Verification items for the finished model (mm, model axes). Round coordinates to 2 decimals unless told otherwise and drop trailing zeros. Write each loop counter-clockwise with the first axis right and the second up, starting at its lowest first coordinate (ties: lowest second). Pieces come first, ordered by that corner, then holes. Notation, with made-up numbers: (79.25, -14) -> (104.25, -14) arc R14 cw to (104.25, 5) -> close; hole circle Ø6 at (61, 29.25). An arc over 180 degrees is marked (long way). Answer as a JSON object with one key per item and string values. Group by question number.
(1) Sectioned sample at A-A on x = -25. Record the cut outline in (y, z).
(2) Gauge pin test, flat ends, axial feed: pin 1 Ø1.5 at (x, z) = (-21, 3.5) entering from -Y; pin 2 Ø1 at (x, z) = (25, 1) entering from -Y; pin 3 Ø2 at (y, z) = (64.5, 4) entering from -X. Record the tip position at first contact, or that the pin passes through.
(3) Scan lines: L1, parallel to Y at x = -17.5, z = 3.1; L2, parallel to X at y = 78, z = 2.75; L3, parallel to Y at x = -4, z = 0.3. Record each from-to range of solid material in increasing order. Write a range as from..to.
(4) Sectioned sample at C-C on x = -12.5. Record the cut outline in (y, z), and give its area (3 significant figures).
(5) Sectioned sample at B-B on y = 82. Record the cut outline in (x, z), and give its area (3 significant figures).
(6) Sectioned sample at D-D on z = 2.6. Count the separate pieces of the cut face and the enclosed holes in it, and give its area (3 significant figures).
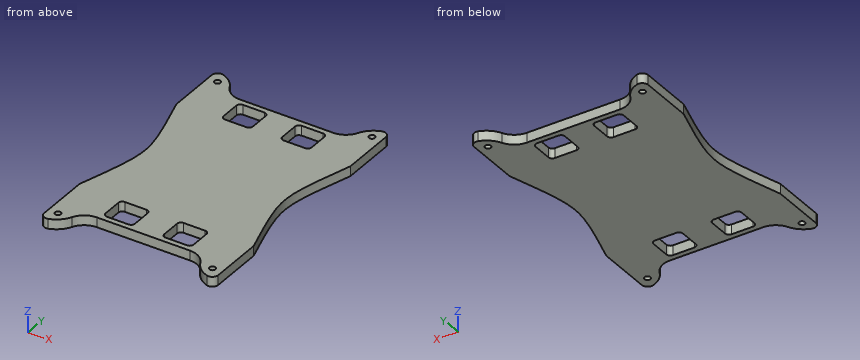
```python
from build123d import *

# Parameters (mm, degrees)
RESSALTO_EXTRUS_O3_DEPTH = 5
ESBO_O4_R                = 1.5
CORTE_EXTRUS_O3_DEPTH    = 10


with BuildPart() as part:
    # Esboço1 → Ressalto-extrusão3 (new body)
    with BuildSketch(Plane.XY):
        with BuildLine():
            Line((-31.851570772, -17.801096987), (-27.063885949, -17.801096987))
            Line((-27.063885949, -17.801096987), (10.936114051, -17.801096987))
            Line((10.936114051, -17.801096987), (15.723798874, -17.801096987))
            ThreePointArc((15.723798874, -17.801096987), (21.039894205, -19.331201448), (24.729153299, -23.4532709))
            ThreePointArc((24.729153299, -23.4532709), (27.934250919, -27.635644423), (32.536114051, -30.202306605))
            ThreePointArc((32.536114051, -30.202306605), (35.210937986, -29.759166326), (36.436114051, -27.340489001))
            Line((36.436114051, -27.340489001), (36.436114051, -17.801096987))
            Line((36.436114051, -17.801096987), (36.436114051, 0.198903013))
            add(Edge.make_bspline(
                [(36.436114051, 75.398903013), (24.729153299, 37.798903013), (36.436114051, 0.198903013)],
                knots=[0, 0, 0, 1, 1, 1], degree=2, weights=[1, 3, 1]))
            Line((36.436114051, 75.398903013), (36.436114051, 93.398903013))
            Line((36.436114051, 93.398903013), (36.436114051, 102.938295027))
            ThreePointArc((36.436114051, 102.938295027), (35.210937986, 105.356972352), (32.536114051, 105.800112631))
            ThreePointArc((32.536114051, 105.800112631), (27.934250919, 103.23345045), (24.729153299, 99.051076926))
            ThreePointArc((24.729153299, 99.051076926), (21.039894205, 94.929007474), (15.723798874, 93.398903013))
            Line((15.723798874, 93.398903013), (10.936114051, 93.398903013))
            Line((10.936114051, 93.398903013), (-27.063885949, 93.398903013))
            Line((-27.063885949, 93.398903013), (-31.851570772, 93.398903013))
            ThreePointArc((-31.851570772, 93.398903013), (-37.167666102, 94.929007474), (-40.856925197, 99.051076926))
            ThreePointArc((-40.856925197, 99.051076926), (-44.062022817, 103.23345045), (-48.663885949, 105.800112631))
            ThreePointArc((-48.663885949, 105.800112631), (-51.338709884, 105.356972352), (-52.563885949, 102.938295027))
            Line((-52.563885949, 102.938295027), (-52.563885949, 93.398903013))
            Line((-52.563885949, 93.398903013), (-52.563885949, 75.398903013))
            add(Edge.make_bspline(
                [(-52.563885949, 75.398903013), (-40.856925197, 37.798903013), (-52.563885949, 0.198903013)],
                knots=[0, 0, 0, 1, 1, 1], degree=2, weights=[1, 3, 1]))
            Line((-52.563885949, 0.198903013), (-52.563885949, -17.801096987))
            Line((-52.563885949, -17.801096987), (-52.563885949, -27.340489001))
            ThreePointArc((-52.563885949, -27.340489001), (-51.338709884, -29.759166326), (-48.663885949, -30.202306605))
            ThreePointArc((-48.663885949, -30.202306605), (-44.062022817, -27.635644423), (-40.856925197, -23.4532709))
            ThreePointArc((-40.856925197, -23.4532709), (-37.167666102, -19.331201448), (-31.851570772, -17.801096987))
        make_face()
    extrude(amount=RESSALTO_EXTRUS_O3_DEPTH)

    # Esboço4 → Corte-extrusão3 (cut)
    with BuildSketch(Plane(origin=(0, 0, 0), x_dir=(-1, 0, 0), z_dir=(0, 0, -1))):
        with Locations((-31.436114051, 99.800112631)):
            Circle(ESBO_O4_R)
        with Locations((47.563885949, 99.800112631)):
            Circle(ESBO_O4_R)
        with Locations((47.563885949, -24.202306605)):
            Circle(ESBO_O4_R)
        with Locations((-31.436114051, -24.202306605)):
            Circle(ESBO_O4_R)
        with BuildLine():
            Line((-12.436114051, 90.598903013), (-1.436114051, 90.598903013))
            ThreePointArc((-1.436114051, 90.598903013), (-0.021900489, 90.013116575), (0.563885949, 88.598903013))
            Line((0.563885949, 88.598903013), (0.563885949, 78.698903013))
            ThreePointArc((0.563885949, 78.698903013), (-0.021900489, 77.284689451), (-1.436114051, 76.698903013))
            Line((-1.436114051, 76.698903013), (-12.436114051, 76.698903013))
            ThreePointArc((-12.436114051, 76.698903013), (-13.850327613, 77.284689451), (-14.436114051, 78.698903013))
            Line((-14.436114051, 78.698903013), (-14.436114051, 88.598903013))
            ThreePointArc((-14.436114051, 88.598903013), (-13.850327613, 90.013116575), (-12.436114051, 90.598903013))
        make_face()
        with BuildLine():
            Line((17.563885949, 90.598903013), (28.563885949, 90.598903013))
            ThreePointArc((28.563885949, 90.598903013), (29.978099511, 90.013116575), (30.563885949, 88.598903013))
            Line((30.563885949, 88.598903013), (30.563885949, 78.698903013))
            ThreePointArc((30.563885949, 78.698903013), (29.978099511, 77.284689451), (28.563885949, 76.698903013))
            Line((28.563885949, 76.698903013), (17.563885949, 76.698903013))
            ThreePointArc((17.563885949, 76.698903013), (16.149672387, 77.284689451), (15.563885949, 78.698903013))
            Line((15.563885949, 78.698903013), (15.563885949, 88.598903013))
            ThreePointArc((15.563885949, 88.598903013), (16.149672387, 90.013116575), (17.563885949, 90.598903013))
        make_face()
        with BuildLine():
            Line((30.563885949, -13.001096987), (30.563885949, -3.101096987))
            ThreePointArc((30.563885949, -3.101096987), (29.978099511, -1.686883425), (28.563885949, -1.101096987))
            Line((28.563885949, -1.101096987), (17.563885949, -1.101096987))
            ThreePointArc((17.563885949, -1.101096987), (16.149672387, -1.686883425), (15.563885949, -3.101096987))
            Line((15.563885949, -3.101096987), (15.563885949, -13.001096987))
            ThreePointArc((15.563885949, -13.001096987), (16.149672387, -14.415310549), (17.563885949, -15.001096987))
            Line((17.563885949, -15.001096987), (28.563885949, -15.001096987))
            ThreePointArc((28.563885949, -15.001096987), (29.978099511, -14.415310549), (30.563885949, -13.001096987))
        make_face()
        with BuildLine():
            Line((0.563885949, -13.001096987), (0.563885949, -3.101096987))
            ThreePointArc((0.563885949, -3.101096987), (-0.021900489, -1.686883425), (-1.436114051, -1.101096987))
            Line((-1.436114051, -1.101096987), (-12.436114051, -1.101096987))
            ThreePointArc((-12.436114051, -1.101096987), (-13.850327613, -1.686883425), (-14.436114051, -3.101096987))
            Line((-14.436114051, -3.101096987), (-14.436114051, -13.001096987))
            ThreePointArc((-14.436114051, -13.001096987), (-13.850327613, -14.415310549), (-12.436114051, -15.001096987))
            Line((-12.436114051, -15.001096987), (-1.436114051, -15.001096987))
            ThreePointArc((-1.436114051, -15.001096987), (-0.021900489, -14.415310549), (0.563885949, -13.001096987))
        make_face()
    extrude(amount=-CORTE_EXTRUS_O3_DEPTH, mode=Mode.SUBTRACT)


solid = part.part
```
Computed values:
{
 "1": {"outline": "(-17.8, 0) -> (-15, 0) -> (-15, 5) -> (-17.8, 5) -> close; (-1.1, 0) -> (76.7, 0) -> (76.7, 5) -> (-1.1, 5) -> close; (90.6, 0) -> (93.4, 0) -> (93.4, 5) -> (90.6, 5) -> close"},
 "2": {"pin 1": "y = -17.8", "pin 2": "y = -24.83", "pin 3": "x = -49.54"},
 "3": {"L1": "-17.8..-15, -1.1..76.7, 90.6..93.4", "L2": "-52.56..-30.44, -15.69..-0.44, 14.31..36.44", "L3": "-17.8..93.4"},
 "4": {"outline": "(-17.8, 0) -> (93.4, 0) -> (93.4, 5) -> (-17.8, 5) -> close", "area": "556 mm2"},
 "5": {"outline": "(-52.56, 0) -> (-30.56, 0) -> (-30.56, 5) -> (-52.56, 5) -> close; (-15.56, 0) -> (-0.56, 0) -> (-0.56, 5) -> (-15.56, 5) -> close; (14.44, 0) -> (36.44, 0) -> (36.44, 5) -> (14.44, 5) -> close", "area": "295 mm2"},
 "6": {"separate pieces": "1", "enclosed holes": "8", "area": "8,820 mm2"}
}
